Read the model definition and answer for the solid it produces. Units are mm, in the model's axes. A direction names the side the tool comes from. Round coordinates to 2 decimals unless told otherwise and drop trailing zeros. Loops run counter-clockwise (first coordinate to the right, second up) from the corner with the lowest first, then second, coordinate; pieces in that order, holes last. Notation, with made-up numbers: M 66,9.25 L 117,9.25 A18 ccw 117,14.25 Z; hole C 82,17.5 d4. An arc over 180 degrees is marked long. Write each question's results on one line, items separated by ' | '.
```python
from build123d import *

# Parameters (mm, degrees)
SKETCH1_W           = 43.18
SKETCH1_H           = 58.42
BOSS_EXTRUDE1_DEPTH = 33.02
SKETCH2_W           = 37.132
SKETCH2_H           = 52.324
CUT_EXTRUDE1_DEPTH  = 25.4
SKETCH2_6_W         = 43.18
SKETCH2_6_H         = 58.42
SKETCH2_6_W_2       = 40.132
SKETCH2_6_H_2       = 55.372
CUT_EXTRUDE3_DEPTH  = 3.81
SKETCH5_W           = 2
SKETCH5_H           = 48.26
BOSS_EXTRUDE2_DEPTH = 38.1
SKETCH6_W           = 26.972
SKETCH6_H           = 48.26
CUT_EXTRUDE4_DEPTH  = 7.62
SKETCH8_W           = 33.02
SKETCH8_H           = 48.26
CUT_EXTRUDE5_DEPTH  = 7.62
SKETCH9_W           = 33.02
SKETCH9_H           = 2.54
BOSS_EXTRUDE3_DEPTH = 2.54
SKETCH11_W          = 33.02
SKETCH11_H          = 5.08
BOSS_EXTRUDE4_DEPTH = 7.62
SKETCH12_W          = 12.7
SKETCH12_H          = 5.08
CUT_EXTRUDE6_DEPTH  = 3.81
FILLET1_R           = 2.54
FILLET2_R           = 2.54
FILLET3_R           = 2.54
FILLET4_R           = 2.54
FILLET5_R           = 1


with BuildPart() as part:
    # Sketch1 → Boss-Extrude1 (new body)
    with BuildSketch(Plane.XY):
        with Locations((6.420456459, 29.21)):
            Rectangle(SKETCH1_W, SKETCH1_H)
    extrude(amount=BOSS_EXTRUDE1_DEPTH)

    # Sketch2 → Cut-Extrude1 (cut)
    with BuildSketch(Plane.XY.offset(33.02)):
        with Locations((6.396456459, 29.21)):
            Rectangle(SKETCH2_W, SKETCH2_H)
    extrude(amount=-CUT_EXTRUDE1_DEPTH, mode=Mode.SUBTRACT)

    # Sketch2<6> → Cut-Extrude3 (cut)
    with BuildSketch(Plane.XY.offset(33.02)):
        with Locations((6.420456459, 29.21)):
            Rectangle(SKETCH2_6_W, SKETCH2_6_H)
        with Locations((6.420456459, 29.21)):
            Rectangle(SKETCH2_6_W_2, SKETCH2_6_H_2, mode=Mode.SUBTRACT)
    extrude(amount=-CUT_EXTRUDE3_DEPTH, mode=Mode.SUBTRACT)

    # Sketch5 → Boss-Extrude2 (add)
    with BuildSketch(Plane(origin=(-12.169543541, 0, 0), x_dir=(0, 0, -1), z_dir=(1, 0, 0))):
        with Locations((-26.21, 29.21)):
            Rectangle(SKETCH5_W, SKETCH5_H)
    extrude(amount=BOSS_EXTRUDE2_DEPTH)

    # Sketch6 → Cut-Extrude4 (cut)
    with BuildSketch(Plane.XY.offset(27.21)):
        with Locations((6.396456459, 29.21)):
            Rectangle(SKETCH6_W, SKETCH6_H)
    extrude(amount=-CUT_EXTRUDE4_DEPTH, mode=Mode.SUBTRACT)

    # Sketch8 → Cut-Extrude5 (cut)
    with BuildSketch(Plane(origin=(0, 0, 0), x_dir=(-1, 0, 0), z_dir=(0, 0, -1))):
        with Locations((-6.420456459, 29.21)):
            Rectangle(SKETCH8_W, SKETCH8_H)
    extrude(amount=-CUT_EXTRUDE5_DEPTH, mode=Mode.SUBTRACT)

    # Sketch9 → Boss-Extrude3 (add)
    with BuildSketch(Plane(origin=(0, 5.08, 0), x_dir=(1, 0, 0), z_dir=(0, 1, 0))):
        with Locations((6.420456459, -1.27)):
            Rectangle(SKETCH9_W, SKETCH9_H)
    extrude(amount=BOSS_EXTRUDE3_DEPTH)

    # Sketch11 → Boss-Extrude4 (add)
    with BuildSketch(Plane.XZ.offset(-53.34)):
        with Locations((6.420456459, 5.08)):
            Rectangle(SKETCH11_W, SKETCH11_H)
    extrude(amount=BOSS_EXTRUDE4_DEPTH)

    # Sketch12 → Cut-Extrude6 (cut)
    with BuildSketch(Plane(origin=(0, 0, 2.54), x_dir=(-1, 0, 0), z_dir=(0, 0, -1))):
        with Locations((-6.420456459, 49.784)):
            Rectangle(SKETCH12_W, SKETCH12_H)
    extrude(amount=-CUT_EXTRUDE6_DEPTH, mode=Mode.SUBTRACT)

    # Fillet1
    # the kernel refuses this fillet: 2.54 mm, written as the material it adds along each edge
    with BuildSketch(Plane(origin=(-12.169543541, 3.048, 33.02), x_dir=(1, 0, 0), z_dir=(0, 0, -1)), Plane(origin=(24.962456459, 55.372, 33.02), x_dir=(-1, 0, 0), z_dir=(0, 0, -1)), Plane(origin=(24.962456459, 3.048, 33.02), x_dir=(0, 1, 0), z_dir=(0, 0, -1))) as fillet1_piece_1:
        with BuildLine():
            CenterArc((FILLET1_R, -FILLET1_R), FILLET1_R, 90, 90)
            Line((0, -FILLET1_R), (0, 0))
            Line((0, 0), (FILLET1_R, 0))
        make_face()
    extrude(amount=31.75)
    with BuildSketch(Plane(origin=(-12.169543541, 55.372, 33.02), x_dir=(1, 0, 0), z_dir=(0, 0, -1))) as fillet1_piece_2:
        with BuildLine():
            CenterArc((FILLET1_R, FILLET1_R), FILLET1_R, 180, 90)
            Line((0, FILLET1_R), (0, 0))
            Line((0, 0), (FILLET1_R, 0))
        make_face()
    extrude(amount=31.75)

    # Fillet2
    fillet2_edges = [part.edges().sort_by_distance(p)[0] for p in [
        (-15.169543541, 58.42, 14.605),
        (28.010456459, 58.42, 14.605),
        (26.486456459, 56.896, 31.115),
        (-13.645543541, 56.896, 31.115),
    ]]
    fillet(fillet2_edges, radius=FILLET2_R)

    # Fillet3
    fillet3_edges = [part.edges().sort_by_distance(p)[0] for p in [
        (-15.169543541, 0, 14.605),
        (-13.645543541, 1.524, 31.115),
    ]]
    fillet(fillet3_edges, radius=FILLET3_R)

    # Fillet4
    fillet4_edges = [part.edges().sort_by_distance(p)[0] for p in [
        (28.010456459, 0, 14.605),
        (26.486456459, 1.524, 31.115),
    ]]
    fillet(fillet4_edges, radius=FILLET4_R)

    # Fillet5
    fillet5_edges = [part.edges().sort_by_distance(p)[0] for p in [
        (-15.169543541, 29.21, 0),
        (6.420456459, 58.42, 0),
        (27.266507683, 57.676051224, 0),
        (-14.425594766, 57.676051224, 0),
        (6.420456459, 0, 0),
        (-14.425594766, 0.743948776, 0),
        (28.010456459, 29.21, 0),
        (27.266507683, 0.743948776, 0),
    ]]
    fillet(fillet5_edges, radius=FILLET5_R)


solid = part.part
```
1. Find section C-C, the plane x = 21.5. Give the vertices of the cut face in (y, z), then the cut area to 3 significant figures.
Completed:
outline: M 0,1 A1 ccw 1,0 L 7.62,0 L 7.62,2.54 L 5.08,2.54 L 5.08,7.62 L 3.05,7.62 L 3.05,33.02 L 1.52,33.02 L 1.52,29.21 L 0,29.21 Z; M 5.08,25.21 L 53.34,25.21 L 53.34,27.21 L 5.08,27.21 Z; M 45.72,2.54 L 53.34,2.54 L 53.34,0 L 57.42,0 A1 ccw 58.42,1 L 58.42,29.21 L 56.9,29.21 L 56.9,33.02 L 55.37,33.02 L 55.37,7.62 L 45.72,7.62 Z | area: 362 mm2
2. Find section B-B, the plane y = 42. Give the vertices of the cut face in (x, z), then the cut area to 3 significant figures.
Completed:
outline: M -15.17,1 A1 ccw -14.17,0 L -10.09,0 L -10.09,7.62 L -12.17,7.62 L -12.17,25.21 L -7.09,25.21 L -7.09,27.21 L -12.17,27.21 L -12.17,33.02 L -13.65,33.02 L -13.65,29.21 L -15.17,29.21 Z; M 19.88,25.21 L 24.96,25.21 L 24.96,7.62 L 22.93,7.62 L 22.93,0 L 27.01,0 A1 ccw 28.01,1 L 28.01,29.21 L 26.49,29.21 L 26.49,33.02 L 24.96,33.02 L 24.96,27.21 L 19.88,27.21 Z | area: 239 mm2
3. Find section D-D, the plane z = 5.5. Give the vertices of the cut face in (x, y).
Completed:
outline: M -15.17,2.54 A2.54 ccw -12.63,0 L 25.47,0 A2.54 ccw 28.01,2.54 L 28.01,55.88 A2.54 ccw 25.47,58.42 L -12.63,58.42 A2.54 ccw -15.17,55.88 Z; hole M -10.09,5.08 L 22.93,5.08 L 22.93,45.72 L -10.09,45.72 Z; hole M 0.07,47.24 L 12.77,47.24 L 12.77,52.32 L 0.07,52.32 Z
4. Given P1, Ø4, axis at x = -4.5, y = 43.5, coming from the -Z side; P2, Ø12, axis at x = -5, y = 36.5, coming from the +Z side; P3, Ø4, axis at y = 17, z = 31.5, coming from the -X side; P4, Ø6, axis at x = 10.5, y = 49, coming from the -Z side, each flat-ended and moving along its own axis, determine where each tip first touches the part or whether it passes through.
Completed:
P1: passes through | P2: stops at z = 27.21 | P3: stops at x = -13.65 | P4: stops at z = 2.54
5. Find section A-A, the plane x = 5. Give the vertices of the cut face in (y, z).
Completed:
outline: M 0,1 A1 ccw 1,0 L 7.62,0 L 7.62,2.54 L 5.08,2.54 L 5.08,7.62 L 3.05,7.62 L 3.05,33.02 L 1.52,33.02 L 1.52,29.21 L 0,29.21 Z; M 45.72,2.54 L 47.24,2.54 L 47.24,6.35 L 52.32,6.35 L 52.32,2.54 L 53.34,2.54 L 53.34,0 L 57.42,0 A1 ccw 58.42,1 L 58.42,29.21 L 56.9,29.21 L 56.9,33.02 L 55.37,33.02 L 55.37,7.62 L 45.72,7.62 Z
6. Find the intervals of material crossed by L1, parallel to Y at x = 10, z = 3; L2, parallel to Y at x = -8.5, z = 11.5; L3, parallel to X at y = 19, z = 13.5, in increasing order.
Completed:
L1: y = 0 to 5.08, 45.72 to 47.24, 52.32 to 58.42 | L2: y = 0 to 3.05, 55.37 to 58.42 | L3: x = -15.17 to -12.17, 24.96 to 28.01
7. Determine the mould class of faces 5 (the face through (22, 5.08, 26)), 6 (the face through (6, 1.524, 31)), 7 (the face through (28.01, 29, 15)) for opening direction X: released by +X, released by -X, zero draft, split by the parting line, or undercut.
Completed:
face 5: undercut | face 6: zero draft | face 7: released by +X
8. Which of the six approach directions +Z, -Z, +X, -X, +Y, -Y give full straight-line access (tool end or side, diameter ignored) to faces 1 (the face through (-10, 29, 25.21)), 2 (the face through (25.762, 56.132, 31.088)), 3 (the face through (-10, 53.34, 26)), 4 (the face through (0.07, 50, 4))?
Completed:
face 1: none | face 2: +Z, +X, +Y | face 3: +Z | face 4: -Z
